Part model, mm, in its own coordinate system. Coordinates: 2 decimals unless noted, no trailing zeros. Write each loop counter-clockwise with the first axis right and the second up, starting at its lowest first coordinate (ties: lowest second). Pieces come first, ordered by that corner, then holes. Notation, with made-up numbers: (64, -40) - (71, -40) arc R23 cw to (71, -20) - close; hole circle Ø7 at (75.25, 49). An arc over 180 degrees is marked (long way). Use a Markdown table: item, result.
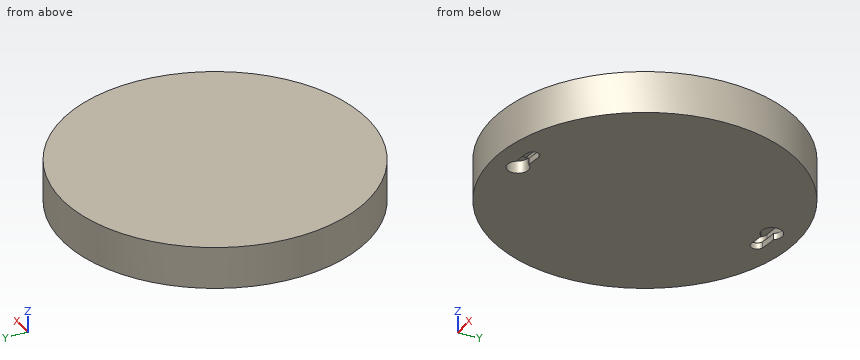
```python
from build123d import *

# Parameters (mm, degrees)
SKETCH002_R        = 36.208774
PAD001_DEPTH       = 10
POCKET001_DEPTH    = 3
POCKET002_DEPTH    = 2
POLARPATTERN_COUNT = 2


with BuildPart() as part:
    # Sketch002 → Pad001 (new body)
    with BuildSketch(Plane.XY):
        Circle(SKETCH002_R)
    extrude(amount=PAD001_DEPTH)

    # Sketch003 (on Face2 of Pad001) → Pocket001 (cut)
    with BuildSketch(Plane(origin=(0, 0, 0), x_dir=(1, 0, 0), z_dir=(0, 0, -1))):
        with BuildLine():
            ThreePointArc((2.048306, 31.433333), (-2.49861, 30.083359), (1.948219, 28.433333))
            ThreePointArc((5.438051, 27.976376), (3.700196, 28.258778), (1.948219, 28.433333))
            ThreePointArc((5.438051, 27.976376), (7.19671, 29.1626), (6.010482, 30.921256))
            ThreePointArc((6.010482, 30.921256), (4.03752, 31.240173), (2.048306, 31.433333))
        make_face()
    pocket001 = extrude(amount=-POCKET001_DEPTH, mode=Mode.SUBTRACT)

    # Sketch004 (on Face2 of Pocket001) → Pocket002 (cut)
    with BuildSketch(Plane(origin=(0, 0, 1.5), x_dir=(1, 0, 0), z_dir=(0, 0, -1))):
        with BuildLine():
            ThreePointArc((0.239614, 32.48849), (-2.48849, 30.239614), (-0.239614, 27.51151))
            Line((-0.239614, 27.51151), (5.484655, 26.960325))
            ThreePointArc((5.484655, 26.960325), (8.21276, 29.209201), (5.963884, 31.937306))
            Line((5.963884, 31.937306), (0.239614, 32.48849))
        make_face()
    pocket002 = extrude(amount=-POCKET002_DEPTH, mode=Mode.SUBTRACT)

    # PolarPattern: Pocket001, Pocket002 ×2 about axis
    polarpattern_axis = Axis((0, 0, 0), (0, 0, -1))
    for i in range(1, POLARPATTERN_COUNT):
        add(pocket001.rotate(polarpattern_axis, i * 360 / POLARPATTERN_COUNT), mode=Mode.SUBTRACT)
        add(pocket002.rotate(polarpattern_axis, i * 360 / POLARPATTERN_COUNT), mode=Mode.SUBTRACT)


solid = part.part
```
Item 1: Band-saw the part on B-B, the plane z = 4.5. Give the cut face in (x, y), then the cut area to 3 significant figures.
From the geometry:
| item | result |
|---|---|
| outline | circle Ø72.42 at (0, 0) |
| area | 4,120 mm^2 |
Item 2: Band-saw the part on D-D, the plane y = 18.5. Give the cut face in (x, z).
From the geometry:
| item | result |
|---|---|
| outline | (-31.13, 0) - (31.13, 0) - (31.13, 10) - (-31.13, 10) - close |
Item 3: Drill centre lines: probe 1 along Y at (x, z) = (0, 1.6); probe 2 along Z at (x, y) = (-2, 32); probe 3 along X at (y, z) = (-30, 0.65) (3 decimals). Where is each one in solid material? Low to high.
From the geometry:
| item | result |
|---|---|
| probe 1 | -36.21 to -32.5, -27.49 to 27.49, 32.5 to 36.21 |
| probe 2 | 0 to 1.5, 3.5 to 10 |
| probe 3 | -20.275 to -2.5, 7.119 to 20.275 |
Item 4: Band-saw the part on C-C, the plane x = -13. Give the cut face in (y, z).
From the geometry:
| item | result |
|---|---|
| outline | (-33.79, 0) - (33.79, 0) - (33.79, 10) - (-33.79, 10) - close |
Item 5: Band-saw the part on A-A, the plane y = 30. Give the cut face in (x, z) (3 decimals).
From the geometry:
| item | result |
|---|---|
| outline | (-20.275, 0) - (-7.119, 0) - (-7.119, 1.5) - (-8.163, 1.5) - (-8.163, 3.5) - (2.5, 3.5) - (2.5, 0) - (20.275, 0) - (20.275, 10) - (-20.275, 10) - close |
Item 6: Drop flat-ended pins along their axis: P1, Ø6, axis at y = -7.5, z = 1.5, coming from the -X side; P2, Ø1, axis at x = -27.5, z = 2.5, coming from the +Y side; P3, Ø4.5, axis at x = 0, y = -30, coming from the -Z side. Give the stop position or say it passes through.
From the geometry:
| item | result |
|---|---|
| P1 | x = -35.93 |
| P2 | y = 24.13 |
| P3 | z = 3.5 |
